Job drawing, mm, ordinate dimensions from the low corner. One solid piece. Round coordinates to 2 decimals unless told otherwise and drop trailing zeros. Loops run counter-clockwise (first coordinate to the right, second up) from the corner with the lowest first, then second, coordinate; pieces in that order, holes last. Notation, with made-up numbers: M 81,78 L 122,78 A13 cw 122,91 Z; hole C 41,-39.5 d3. An arc over 180 degrees is marked long. Use one line per item in the form item = value. Start each with the question number.
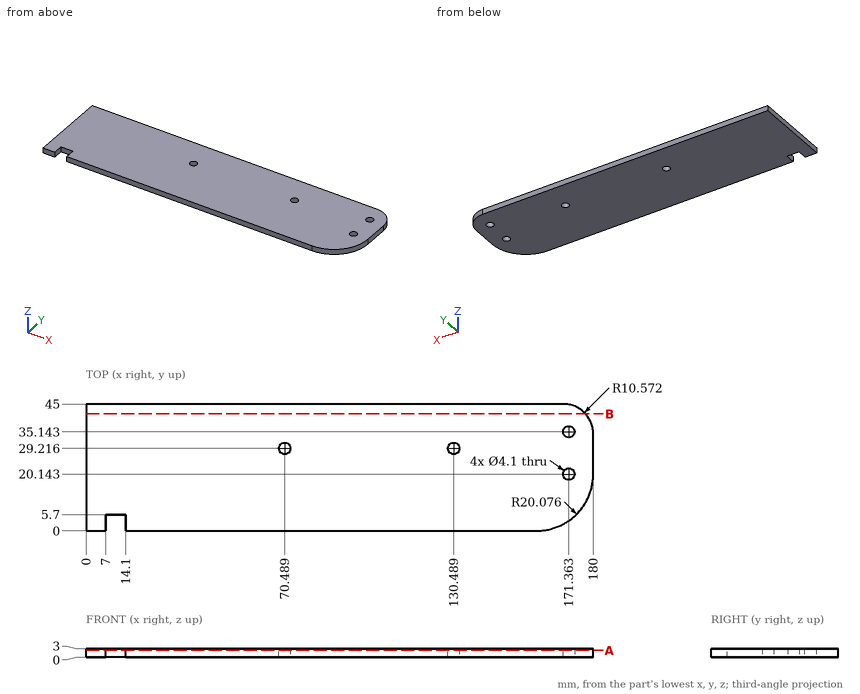
Q1. Saw through at B-B (y = 41.5). Give the cut face in (x, z), and give its area (3 significant figures).
Q2. Saw through at A-A (z = 2.4). Give the number of separate pieces and of enclosed holes in the cut face, and give its area (3 significant figures).
Q3. Wall check: probe 1 along X at (y, z) = (28, 1); probe 2 along Y at (x, z) = (70.5, 2.6); probe 3 along X at (y, z) = (30, 0.3) (1 decimal). Give the ranges that are in metal, low to high.
Q4. Drop flat-ended pins along their axis: P1, Ø2.5, axis at x = 70.49, y = 29.22, coming from the -Z side; P2, Ø0.9, axis at y = 2.5, z = 2, coming from the +X side; P3, Ø1.5, axis at x = 12.5, z = 1.5, coming from the -Y side. Give the stop position or say it passes through.
Filled in:
q1.outline = M 0,0 L 177.29,0 L 177.29,3 L 0,3 Z
q1.area = 532 mm²
q2.separate_pieces = 1
q2.enclosed_holes = 4
q2.area = 7,900 mm²
q3.probe_1 = 0 to 68.84, 72.14 to 128.84, 132.14 to 180
q3.probe_2 = 0 to 27.17, 31.27 to 45
q3.probe_3 = 0 to 68.6, 72.4 to 128.6, 132.4 to 180
q4.P1 = through
q4.P2 = 170.4
q4.P3 = 5.7
